Geometry: final body of the model. Coordinates: model frame, mm. A direction names the side the tool comes from. Coordinates: 2 decimals unless noted, no trailing zeros. Write each loop counter-clockwise with the first axis right and the second up, starting at its lowest first coordinate (ties: lowest second). Pieces come first, ordered by that corner, then holes. Notation, with made-up numbers: (88, 14.5) -> (104, 14.5) arc R21 cw to (104, 51.5) -> close; hole circle Ø1 at (42, 19). An arc over 180 degrees is marked (long way). One line per item, written item: value. Start each with the question number.
from build123d import *

# Parameters (mm, degrees)
F0_W     = 273.05
F0_H     = 114.3
F1_DEPTH = 19.05
F2_R     = 38.1
F3_DEPTH = 25.4
F5_DEPTH = 25.4
F6_DEPTH = 25.4
F7_DEPTH = 25.4


with BuildPart() as f1:
    # F0 (on Front) → F1 (new body)
    with BuildSketch(Plane.XZ):
        with Locations((136.525, 57.15)):
            Rectangle(F0_W, F0_H)
    extrude(amount=F1_DEPTH)

    # F2 (on Front) → F3 (cut)
    with BuildSketch(Plane.XZ):
        with Locations((50.8, 47.625)):
            Circle(F2_R)
        with Locations((222.25, 47.625)):
            Circle(F2_R)
    extrude(amount=F3_DEPTH, mode=Mode.SUBTRACT)

    # F4 (on Front) → F5 (cut)
    with BuildSketch(Plane.XZ):
        with BuildLine():
            Line((177.8, 114.074679), (95.25, 114.074679))
            Line((95.25, 114.074679), (95.25, 62.23))
            ThreePointArc((95.25, 62.23), (98.597769, 54.147769), (106.68, 50.8))
            Line((106.68, 50.8), (166.37, 50.8))
            ThreePointArc((166.37, 50.8), (174.452231, 54.147769), (177.8, 62.23))
            Line((177.8, 62.23), (177.8, 114.074679))
        make_face()
    extrude(amount=-F5_DEPTH, mode=Mode.SUBTRACT)

    # F4 (on Front) → F6 (cut)
    with BuildSketch(Plane.XZ):
        with BuildLine():
            Line((177.8, 114.074679), (95.25, 114.074679))
            Line((95.25, 114.074679), (95.25, 62.23))
            ThreePointArc((95.25, 62.23), (98.597769, 54.147769), (106.68, 50.8))
            Line((106.68, 50.8), (166.37, 50.8))
            ThreePointArc((166.37, 50.8), (174.452231, 54.147769), (177.8, 62.23))
            Line((177.8, 62.23), (177.8, 114.074679))
        make_face()
    extrude(amount=F6_DEPTH, mode=Mode.SUBTRACT)

    # F4 (on Front) → F7 (cut)
    with BuildSketch(Plane.XZ):
        with BuildLine():
            Line((177.8, 114.074679), (95.25, 114.074679))
            Line((95.25, 114.074679), (95.25, 62.23))
            ThreePointArc((95.25, 62.23), (98.597769, 54.147769), (106.68, 50.8))
            Line((106.68, 50.8), (166.37, 50.8))
            ThreePointArc((166.37, 50.8), (174.452231, 54.147769), (177.8, 62.23))
            Line((177.8, 62.23), (177.8, 114.074679))
        make_face()
    extrude(amount=-F7_DEPTH, mode=Mode.SUBTRACT)


solid = f1.part
Q1. First-contact query: P1, Ø1.5, axis at y = -2.5, z = 95, coming from the -X side. Flat tip, straight axial feed; report the tip coordinate or a pass-through.
Q2. Draft query along X for faces 3 (the flat face through (135, -9, 0)), 4 (the flat face through (137, -9, 114.075)), 5 (the flat face through (273.05, -9, 56)). Return one class per face: pulls with the +X half, pulls with the -X half, needs draft (parallel to the pull), parting line crosses it, or undercut.
Q3. Cut plane B-B on z = 100.5. Output: boundary loops of the cut face in (x, y).
Q4. Access query for faces 1 (the flat face through (136, -9, 50.8)), 2 (the flat face through (135, -9, 114.3)). Directions: +Z, -Z, +X, -X, +Y, -Y. A direction counts if a zero-diameter tool reaches every point of the face in a straight line with its end or side. Return the directions, or none.
Q5. Line query: L1, parallel to X at y = -15.25, z = 47; L2, parallel to Z at x = 162.5, y = -3.5; L3, parallel to Z at x = 222.25, y = -8.5 (3 decimals). Output: solid intervals per line, ascending. Write a range as from..to.
Q6. Cut plane A-A on x = 50.8. Output: boundary loops of the cut face in (y, z) (3 decimals).
Q7. Cut plane D-D on z = 12. Output: boundary loops of the cut face in (x, y).
Q8. Cut plane C-C on y = -15.5. Output: boundary loops of the cut face in (x, z) (3 decimals).
Solution:
1. P1: x = 0
2. face 3: needs draft
2. face 4: undercut
2. face 5: pulls with the +X half
3. outline: (0, -19.05) -> (95.25, -19.05) -> (95.25, 0) -> (0, 0) -> close; (177.8, -19.05) -> (273.05, -19.05) -> (273.05, 0) -> (177.8, 0) -> close
4. face 1: +Y, -Y
4. face 2: +Z, +X, -X, +Y, -Y
5. L1: 0..12.71, 88.89..184.16, 260.34..273.05
5. L2: 0..50.8, 114.07..114.3
5. L3: 0..9.525, 85.725..114.3
6. outline: (-19.05, 0) -> (0, 0) -> (0, 9.525) -> (-19.05, 9.525) -> close; (-19.05, 85.725) -> (0, 85.725) -> (0, 114.3) -> (-19.05, 114.3) -> close
7. outline: (0, -19.05) -> (37.29, -19.05) -> (37.29, 0) -> (0, 0) -> close; (64.31, -19.05) -> (208.74, -19.05) -> (208.74, 0) -> (64.31, 0) -> close; (235.76, -19.05) -> (273.05, -19.05) -> (273.05, 0) -> (235.76, 0) -> close
8. outline: (0, 0) -> (273.05, 0) -> (273.05, 114.3) -> (0, 114.3) -> close; hole circle Ø76.2 at (50.8, 47.625); hole (95.25, 62.23) arc R11.43 ccw to (106.68, 50.8) -> (166.37, 50.8) arc R11.43 ccw to (177.8, 62.23) -> (177.8, 114.075) -> (95.25, 114.075) -> close; hole circle Ø76.2 at (222.25, 47.625)
